```python
from build123d import *

# Parameters (mm, degrees)
SKETCH2_R           = 16.66875
SKETCH2_R_2         = 12.954
SKETCH2_R_3         = 11.1125
BOSS_EXTRUDE1_DEPTH = 3.175
SKETCH2_3_R         = 12.954
SKETCH2_3_R_2       = 11.1125
BOSS_EXTRUDE2_DEPTH = 3.5433


with BuildPart() as part:
    # Sketch2 → Boss-Extrude1 (new body, symmetric)
    with BuildSketch(Plane(origin=(0, 0, 0), x_dir=(1, 0, 0), z_dir=(0, 1, 0))):
        Circle(SKETCH2_R)
        Circle(SKETCH2_R_2, mode=Mode.SUBTRACT)
        Circle(SKETCH2_R_2)
        Circle(SKETCH2_R_3, mode=Mode.SUBTRACT)
    extrude(amount=BOSS_EXTRUDE1_DEPTH, both=True)

    # Sketch2_3 → Boss-Extrude2 (add, symmetric)
    with BuildSketch(Plane(origin=(0, 0, 0), x_dir=(1, 0, 0), z_dir=(0, 1, 0))):
        Circle(SKETCH2_3_R)
        Circle(SKETCH2_3_R_2, mode=Mode.SUBTRACT)
    extrude(amount=BOSS_EXTRUDE2_DEPTH, both=True)


solid = part.part
```
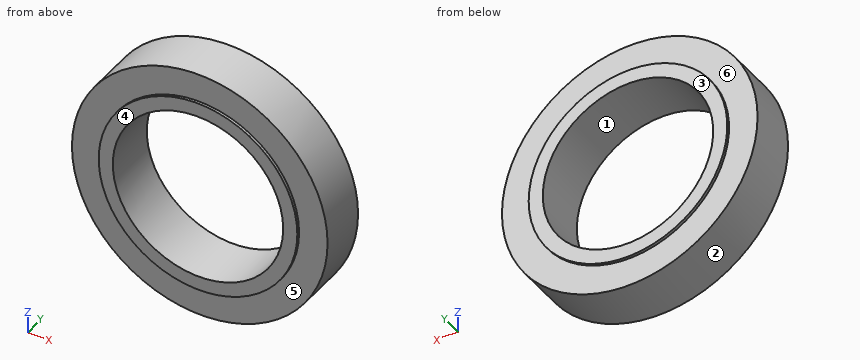
Work out the finished part from the listing and answer in its coordinate system (mm). Face numbers are marked on the shaded views. A direction names the side the tool comes from. Coordinates: 2 decimals unless noted, no trailing zeros. Write each loop counter-clockwise with the first axis right and the second up, starting at its lowest first coordinate (ties: lowest second). Pieces come first, ordered by that corner, then holes.
Q1. A cutting plane is placed at D-D, the plane z = 11.5. Give the vertices of the cut face in (x, y) (3 decimals).
Q2. Which of the six approach directions +Z, -Z, +X, -X, +Y, -Y give full straight-line access (tool end or side, diameter ignored) to the marked faces 4, 5 and 6?
Q3. Determine the mould class of the marked faces 1, 2 and 3 for opening direction X: released by +X, released by -X, zero draft, split by the parting line, or undercut.
Q4. A cutting plane is placed at C-C, the plane y = -0.5. Give the vertices of the cut face in (x, z) (1 decimal).
Q5. Find the intervals of material crossed by line 1 (Z direction, x = 0, y = 1.25); line 2 (Y direction, x = -2, z = -14.5) (3 decimals), in increasing order.
Q6. Each of these flat-tipped pins is pushed along its axis until it touches: pin 1 Ø6 at (x, z) = (4, -6.5) entering from -Y; pin 2 Ø1 at (y, z) = (0, 11) entering from -X; pin 3 Ø3 at (y, z) = (0.5, 5.5) entering from +X. Where does it stop, or does it pass through?
Findings below:
1. outline: (-12.066, -3.175) - (-5.963, -3.175) - (-5.963, -3.543) - (5.963, -3.543) - (5.963, -3.175) - (12.066, -3.175) - (12.066, 3.175) - (5.963, 3.175) - (5.963, 3.543) - (-5.963, 3.543) - (-5.963, 3.175) - (-12.066, 3.175) - close
2. face 4: +Z, -Z, +X, -X, -Y
2. face 5: -Y
2. face 6: +Y
3. face 1: undercut
3. face 2: split by the parting line
3. face 3: zero draft
4. outline: circle Ø33.3 at (0, 0); hole circle Ø22.2 at (0, 0)
5. line 1: z = -16.67 to -11.11, 11.11 to 16.67
5. line 2: y = -3.175 to 3.175
6. pin 1: passes through
6. pin 2: stops at x = -12.95
6. pin 3: stops at x = 16.18
